Geometry: final body of the model. Coordinates: model frame, mm. Give positions to 0.01 mm unless a question says otherwise; leave off trailing zeros. Loops run counter-clockwise (first coordinate to the right, second up) from the corner with the lowest first, then second, coordinate; pieces in that order, holes last. Notation, with made-up numbers: (67, 72) -> (72, 72) arc R18 cw to (72, 101) -> close; hole circle Ø2 at (-27.75, -0.5). An arc over 180 degrees is marked (long way). Answer in a Markdown table with one row per item. Add a question column.
Autodesk Inventor part; units mm, degrees
ref_plane "YZ Plane" through (0, 0, 0) normal (1, 0, 0) x (0, 1, 0)
ref_plane "XZ Plane" through (0, 0, 0) normal (0, 1, 0) x (-1, 0, 0)
ref_plane "XY Plane" through (0, 0, 0) normal (0, 0, 1) x (1, 0, 0)
sketch "Sketch1" plane through (0, 0, 0) normal (0, 0, 1) x (1, 0, 0)
  circle A0 centre (0, 0) radius 1
  circle A1 centre (47.0377, -0.0423) radius 1
  arc A2 (2.2923, 0.9976) -> (2.2904, -1.0021) centre (0, 0) ccw
  arc A3 (44.7455, -1.0402) -> (44.7473, 0.9598) centre (47.0377, -0.0423) ccw
  line L0 (0, -2) -> (0, 1)
  line L1 (48.4179, 2.0423) -> (48.671, 2.0423)
  line L2 (48.671, -1.9577) -> (48.6442, -1.9577)
  line L3 (48.671, 2.0423) -> (48.671, 1.8505)
  line L4 (48.671, -1.935) -> (48.671, -1.9577)
  line L5 (0, 1) -> (0.0018, 1)
  line L6 (2.2923, 0.9976) -> (44.7473, 0.9598)
  line L7 (47.0404, -1.0422) -> (47.0368, -1.0423)
  line L8 (44.7455, -1.0402) -> (2.2904, -1.0021)
  dimension "d0" = 2
  dimension "d1" = 2
  dimension "d2" = 5
  dimension "d3" = 5
  dimension "d5" = 4
extrude "Extrusion1" add sketch "Sketch1" along normal blind 1.4 contours L6 A3 L8 A2
sketch "Sketch2" plane through (0, 0, 0) normal (0, 0, -1) x (-1, 0, 0)
  point P0 (0, 0)
sketch "Sketch3" plane through (44.7455, -1.0402, 0) normal (-0.0008981, -0.9999996, 0) x (0.9999996, -0.0008981, 0)
  point P0 (-44.7464, 0)
sketch "Sketch4" plane through (44.7455, -1.0402, 0) normal (-0.0008981, -0.9999996, 0) x (0.9999996, -0.0008981, 0)
  line L0 (-44.7455, 0) -> (-24.7455, 0)
  line L1 (-24.7455, 0) -> (-24.7455, 4.8561)
  line L2 (-24.7455, -1.4779) -> (7.1983, -1.4779)
  line L3 (7.1983, -1.4779) -> (7.1983, 5.595)
  line L4 (7.1983, 5.595) -> (-24.7455, 5.595)
  line L5 (-24.7455, 5.595) -> (-24.7455, -1.4779)
  point P0 (-44.7464, 0)
  dimension "d8" = 20
extrude "Extrusion2" cut sketch "Sketch4" along normal mid plane 10
mirror "Mirror1" about plane through (20, -1.018, 5.595) normal (0.9999996, -0.0008981, 0)
properties part number "Restrain_Pin_Pinky_1"
(1) Cut plane B-B on z = 0.25. Return the cut outline in (x, y), then the cut area to 3 significant figures.
(2) Material intervals for line 1 along X through (y, z) = (0, 1.2); line 2 along Y through (x, z) = (0, 0.35); line 3 along X through (y, z) = (0.7, 0.6), sorted ascending. Write a range as from..to.
(3) Draft query along X for faces 1 (the cylindrical face through (-2.5, -0.09, 0.69)), 2 (the flat face through (20, 0, 0)). Return one class per face: +X half, -X half, draft (parallel to the pull), parting line (faces both ways), or undercut.
(4) Cut plane A-A on x = 0. Return the cut outline in (y, z), then the cut area to 3 significant figures.
(5) Cut plane C-C on x = 10.5. Return the cut outline in (y, z), then the cut area to 3 significant figures.
Answer list:
| question | item | result |
|---|---|---|
| 1 | outline | (2.29, -1) -> (20, -1.02) -> (37.71, -1.03) arc R2.5 ccw (long way) to (37.71, 0.97) -> (20, 0.98) -> (2.29, 1) arc R2.5 ccw (long way) to start; hole circle Ø2 at (0, 0); hole circle Ø2 at (40, -0.04) |
| 1 | area | 103 mm² |
| 2 | line 1 | x = -2.5..-1, 1..39, 41..42.5 |
| 2 | line 2 | y = -2.5..-1, 1..2.5 |
| 2 | line 3 | x = -2.4..-0.71, 0.71..39.32, 40.68..42.39 |
| 3 | face 1 | undercut |
| 3 | face 2 | draft |
| 4 | outline | (-2.5, 0) -> (-1, 0) -> (-1, 1.4) -> (-2.5, 1.4) -> close; (1, 0) -> (2.5, 0) -> (2.5, 1.4) -> (1, 1.4) -> close |
| 4 | area | 4.20 mm² |
| 5 | outline | (-1.01, 0) -> (0.99, 0) -> (0.99, 1.4) -> (-1.01, 1.4) -> close |
| 5 | area | 2.80 mm² |
